Read the model definition and answer for the solid it produces. Units are mm, in the model's axes. A direction names the side the tool comes from. Coordinates: 2 decimals unless noted, no trailing zeros. Order: outer loops, then holes, each group sorted by start corner. A loop starts at its lowest first (then second) coordinate and runs counter-clockwise, first axis right, second up. Notation, with made-up numbers: (-21.75, 45) -> (-4.75, 45) arc R23 ccw to (-4.75, 73) -> close; hole circle Ø7 at (32, 29). An arc over 180 degrees is marked (long way). Return JSON: item names as keys, results as strings. Group by question number.
```python
from build123d import *

# Parameters (mm, degrees)
BOSS_EXTRUDE1_DEPTH = 25.4
CUT_EXTRUDE1_REACH  = 63.561
SKETCH2_R           = 4.7625


with BuildPart() as part:
    # Sketch1 → Boss-Extrude1 (new body)
    with BuildSketch(Plane.XY):
        Polygon((0, 0), (25.4, 0), (25.4, 23.749), (50.8, 23.749), (50.8, 30.099), (19.05, 30.099), (19.05, 6.35), (0, 6.35), align=None)
    extrude(amount=BOSS_EXTRUDE1_DEPTH)

    # Mirror1: part across plane


with BuildPart() as part_1:
    add(part.part)
    add(part.part.mirror(Plane(origin=(0, 6.35, 25.4), x_dir=(0, 0, 1), z_dir=(1, 0, 0))))

    # Sketch2 → Cut-Extrude1 (cut, up to next)
    with BuildSketch(Plane(origin=(0, 6.35, 0), x_dir=(1, 0, 0), z_dir=(0, 1, 0)), mode=Mode.PRIVATE) as cut_extrude1_sk1:
        with Locations(Location((0, -12.7, 0), (0, 0, 180))):
            Circle(SKETCH2_R)
    cut_extrude1_tool1 = extrude(cut_extrude1_sk1.sketch, amount=-CUT_EXTRUDE1_REACH, mode=Mode.PRIVATE) & part_1.part
    add(cut_extrude1_tool1.solids().sort_by_distance((0, 6.35, 12.7))[0], mode=Mode.SUBTRACT)


solid = part_1.part
```
1. Find section A-A on x = 0. Determine the outline of the cut face in (y, z).
2. Find section D-D on z = 20. Determine the outline of the cut face in (x, y).
3. Straight lines are drawn through the part: L1, parallel to X at y = 12.5, z = 19; L2, parallel to Z at x = 0, y = 2.5; L3, parallel to Y at x = -35, z = 7.75. For each, find the intervals that lie inside material, in ascending order.
4. Given pin 1 (8 mm diameter, centred on y = 5.5, z = 12, fed in from -X); pin 2 (1.5 mm diameter, centred on x = 40, z = 15, fed in from -Y); pin 3 (7.5 mm diameter, centred on x = 1, z = 18.5, fed in from +Y), each flat-ended and moving along its own axis, determine where each tip first touches the part or whether it passes through.
5. Find section B-B on z = 12.7. Determine the outline of the cut face in (x, y).
6. Which of the six approach directions +Z, -Z, +X, -X, +Y, -Y give full straight-line access (tool end or side, diameter ignored) to faces 1 (the face through (-25.4, 12, 13)), 2 (the face through (4, 6.35, 9.7)), 3 (the face through (38, 23.749, 13))?
7. Find section C-C on y = 22. Determine the outline of the cut face in (x, z).
8. For a pull along X with two mould halves and no side action, classify faces 4 (the face through (50.8, 27, 13)), 5 (the face through (-19.05, 18, 13)), 6 (the face through (1, 5, 0)) as released by +X, released by -X, zero draft, split by the parting line, or undercut.
Result:
{
 "1": {"outline": "(0, 0) -> (6.35, 0) -> (6.35, 7.94) -> (0, 7.94) -> close; (0, 17.46) -> (6.35, 17.46) -> (6.35, 25.4) -> (0, 25.4) -> close"},
 "2": {"outline": "(-50.8, 23.75) -> (-25.4, 23.75) -> (-25.4, 0) -> (25.4, 0) -> (25.4, 23.75) -> (50.8, 23.75) -> (50.8, 30.1) -> (19.05, 30.1) -> (19.05, 6.35) -> (-19.05, 6.35) -> (-19.05, 30.1) -> (-50.8, 30.1) -> close"},
 "3": {"L1": "-25.4 to -19.05, 19.05 to 25.4", "L2": "0 to 7.94, 17.46 to 25.4", "L3": "23.75 to 30.1"},
 "4": {"pin 1": "x = -25.4", "pin 2": "y = 23.75", "pin 3": "y = 6.35"},
 "5": {"outline": "(-50.8, 23.75) -> (-25.4, 23.75) -> (-25.4, 0) -> (-4.76, 0) -> (-4.76, 6.35) -> (-19.05, 6.35) -> (-19.05, 30.1) -> (-50.8, 30.1) -> close; (4.76, 0) -> (25.4, 0) -> (25.4, 23.75) -> (50.8, 23.75) -> (50.8, 30.1) -> (19.05, 30.1) -> (19.05, 6.35) -> (4.76, 6.35) -> close"},
 "6": {"face 1": "+Z, -Z, -X, -Y", "face 2": "+Z, -Z, +Y", "face 3": "+Z, -Z, +X, -Y"},
 "7": {"outline": "(-25.4, 0) -> (-19.05, 0) -> (-19.05, 25.4) -> (-25.4, 25.4) -> close; (19.05, 0) -> (25.4, 0) -> (25.4, 25.4) -> (19.05, 25.4) -> close"},
 "8": {"face 4": "released by +X", "face 5": "undercut", "face 6": "zero draft"}
}
